Autodesk Inventor part; units mm, degrees
ref_plane "YZ Plane" through (0, 0, 0) normal (1, 0, 0) x (0, 1, 0)
ref_plane "XZ Plane" through (0, 0, 0) normal (0, 1, 0) x (-1, 0, 0)
ref_plane "XY Plane" through (0, 0, 0) normal (0, 0, 1) x (1, 0, 0)
sketch "Sketch2" plane through (0, 0, 0) normal (1, 0, 0) x (0, 1, 0)
  line L0 (0, 10.4889) -> (0, -1.7482)
  line L1 (-17.7123, 0) -> (21.1316, 0)
  line L2 (13, 0) -> (13, 2)
  arc A0 (-7.4177, 7.7315) -> (-8.5, 2.0042) centre (-8.6583, 5) ccw
  line L3 (-8.5, 2.0042) -> (-8.5, 0)
  line L4 (7, 3) -> (8.7479, 6.0075)
  arc A1 (13, 2) -> (8.7479, 6.0075) centre (11.3417, 4.5) ccw
  circle A2 centre (11.3417, 4.5) radius 1.3
  circle A3 centre (-8.6583, 5) radius 1.3
  line L5 (7, 3) -> (3, 3)
  line L6 (3, 3) -> (-7.4177, 7.7315)
  dimension "d0" = 21.5
  dimension "d2" = 3
  dimension "d3" = 2
  dimension "d6" = 3
  dimension "d7" = 4.5
  dimension "d8" = 1.6583
  dimension "d9" = 5
  dimension "d10" = 20
  dimension "d16" = 3
  dimension "d17" = 2.6
  dimension "d30" = 13
  dimension "d31" = 4
  dimension "d32" = 6
extrude "Extrusion1" add sketch "Sketch2" along normal mid plane 12
fillet "Fillet1" radius 1 2 edges at (6, 2.25, 0) (-6, 2.25, 0)
shell "Shell1" thickness 1 removed faces 9 at (2, -9.3053, 7.9294) at (2, 8.1653, 5.005) at (2, 13.3771, 2.2962) at (1.6667, -8.5, 1.3361) at (-1.6667, 13, 1.3333) at (2, 12.6249, 4.2915) at (2, -7.3751, 4.7915) at (-2, -3.9452, 6.1543) at (-2, 4.3333, 3)
sketch "Sketch4" plane through (0, 0, 0) normal (1, 0, 0) x (0, 1, 0)
  arc A0 (-11.4544, 3.4791) -> (-8.5, 1) centre (-8.5, 4) ccw
  arc A1 (-12.4392, 3.3054) -> (-8.5, 0) centre (-8.5, 4) ccw
  line L0 (-12.4392, 3.3054) -> (-11.4544, 3.4791)
  line L1 (-8.5, 1) -> (-8.5, 0)
  line L2 (-8.5, 0) -> (-8.5, 1)
  line L3 (-8.5, 0) -> (13, 0)
  line L4 (13, 1) -> (-8.5, 1)
  dimension "d40" = 3
  dimension "d42" = 1
  dimension "d43" = 80
extrude "Extrusion3" add sketch "Sketch4" along normal mid plane 10
fillet "Fillet2" radius 0.5 2 edges at (-5, 2.25, 1) (5, 2.25, 1)
properties part number "Linkage for 45 degree hinge" material "Steel"
Geometry: final body of the model. Coordinates: model frame, mm. A direction names the side the tool comes from. Coordinates: 2 decimals unless noted, no trailing zeros. Order: outer loops, then holes, each group sorted by start corner. A loop starts at its lowest first (then second) coordinate and runs counter-clockwise, first axis right, second up. Notation, with made-up numbers: (-2, -25) - (18, -25) arc R14 cw to (18, -13) - close; hole circle Ø5 at (57.25, -31.75). An arc over 180 degrees is marked (long way). Return JSON: item names as keys, results as strings. Group by question number.
1. Pin query (flat end, axial travel): pin 1 (2 mm diameter, centred on y = 2, z = 5, fed in from +X); pin 2 (1 mm diameter, centred on y = -10.5, z = 1, fed in from -X); pin 3 (4 mm diameter, centred on x = 1.5, z = 4, fed in from -Y); pin 4 (0.6 mm diameter, centred on x = -2.5, z = 1, fed in from +Y). Return the tip coordinate at first contact, or that it passes through.
2. Pull-direction query (Z, two-part tool) for faces 6 (the face through (5.507, 11.942, 3.347)), 7 (the face through (0, 2, 1)), 8 (the face through (-5, -10, 1)); classes: pulls with the +Z half, pulls with the -Z half, needs draft (parallel to the pull), parting line crosses it, or undercut.
3. Cut plane D-D (z = 6.75). Output: boundary loops of the cut face in (x, y), plus the area to 3 significant figures.
4. Cut plane A-A (z = 5.25). Count the separate pieces of the cut face and the enclosed holes in it, plus the area to 3 significant figures.
5. Cut plane B-B (x = -3.5). Output: boundary loops of the cut face in (y, z), plus the area to 3 significant figures.
6. Set-up query: faces 1 (the face through (-0.07, -11.95, 3.39)), 2 (the face through (-5.5, 5, 3)), 3 (the face through (5, -10, 1)), 4 (the face through (-5, 1, 3)), 5 (the face through (5.51, -7.46, 4.5)). Return all of +Z, -Z, +X, -X, +Y, -Y with unobstructed straight access to the full face (end or side cutting, diameter ignored); none if empty.
7. Material intervals for line 1 along X through (y, z) = (12.75, 1.75); line 2 along Z through (x, y) = (-1, -0.25); line 3 along Y through (x, z) = (0, 3.25), sorted ascending. Write a range as [from, to].
8. Cut plane C-C (y = 11.75). Output: boundary loops of the cut face in (x, z), plus the area to 3 significant figures.
Resolved:
{
 "1": {"pin 1": "passes through", "pin 2": "stops at x = -5", "pin 3": "stops at y = -12.44", "pin 4": "stops at y = 13"},
 "2": {"face 6": "undercut", "face 7": "pulls with the +Z half", "face 8": "needs draft"},
 "3": {"outline": "(-6, -11.1) - (-5, -11.1) - (-5, -5.26) - (-6, -5.26) - close; (-6, 9.36) - (-5, 9.36) - (-5, 13.33) - (-6, 13.33) - close; (5, -11.1) - (6, -11.1) - (6, -5.26) - (5, -5.26) - close; (5, 9.36) - (6, 9.36) - (6, 13.33) - (5, 13.33) - close", "area": "19.6 mm²"},
 "4": {"separate pieces": "8", "enclosed holes": "0", "area": "21.9 mm²"},
 "5": {"outline": "(-12.44, 3.31) arc R4 ccw to (-8.5, 0) - (13, 0) - (13, 1) - (-8.5, 1) arc R3 cw to (-11.45, 3.48) - close", "area": "26.4 mm²"},
 "6": {"face 1": "+Z, +X, -X, -Y", "face 2": "+Z, +X, -X", "face 3": "-Z, +X, -Y", "face 4": "+Z, +Y", "face 5": "+X, -X"},
 "7": {"line 1": "x = [-6, -5], [5, 6]", "line 2": "z = [0, 1]", "line 3": "y = [-12.43, -11.4]"},
 "8": {"outline": "(-6, 1) arc R1 ccw to (-5, 0) - (5, 0) arc R1 ccw to (6, 1) - (6, 3.27) - (5, 3.27) - (5, 1.5) arc R0.5 cw to (4.5, 1) - (-4.5, 1) arc R0.5 cw to (-5, 1.5) - (-5, 3.27) - (-6, 3.27) - close; (-6, 5.73) - (-5, 5.73) - (-5, 7.47) - (-6, 7.47) - close; (5, 5.73) - (6, 5.73) - (6, 7.47) - (5, 7.47) - close", "area": "19.7 mm²"}
}
